from build123d import *

# Parameters (mm, degrees)
SKETCH_1_R = 1.5875


with BuildPart() as part:
    # 草图1 → 旋转1 (revolve)
    with BuildSketch(Plane.XY, mode=Mode.PRIVATE) as revolve_1_sk:
        with BuildLine():
            Line((42.275, 6.35), (42.275, 4.407946167))
            ThreePointArc((42.275, 4.407946167), (42.708118322, 3.857882219), (42.8625, 3.175))
            ThreePointArc((42.8625, 3.175), (42.708118322, 2.492117781), (42.275, 1.942053833))
            Line((42.275, 1.942053833), (42.275, 0))
            Line((42.275, 0), (44.45, 0))
            Line((44.45, 0), (44.45, 6.1))
            Line((44.45, 6.1), (44.45, 6.35))
            Line((44.45, 6.35), (42.275, 6.35))
        make_face()
        with BuildLine():
            Line((40.275, 6.35), (38.1, 6.35))
            Line((38.1, 6.35), (38.1, 6.1))
            Line((38.1, 6.1), (38.1, 0))
            Line((38.1, 0), (40.275, 0))
            Line((40.275, 0), (40.275, 1.942053833))
            ThreePointArc((40.275, 1.942053833), (39.6875, 3.175), (40.275, 4.407946167))
            Line((40.275, 4.407946167), (40.275, 6.35))
        make_face()
        with Locations((41.275, 3.175)):
            Circle(SKETCH_1_R)
    revolve(revolve_1_sk.sketch.rotate(Axis((0, 13.35, 0), (0, 1, 0)), 90), axis=Axis((0, 13.35, 0), (0, 1, 0)))


solid = part.part
The model under review builds one solid part; all positions refer to its coordinate system, in mm. Round coordinates to 2 decimals unless told otherwise and drop trailing zeros. Return JSON: item names as keys, results as strings.
(1) The part is to be moulded in two halves that separate along Z. For faces 1 (the cylindrical face through (-30, 3.2, 32.8)), 2 (the flat face through (30, 0, -24)), 3 (the cylindrical face through (-12.098, 5.393, -38.415)), say which applies: released by +Z, released by -Z, zero draft, split by the parting line, or undercut.
Solved:
{"face 1": "split by the parting line", "face 2": "zero draft", "face 3": "undercut"}
(2) For line 1 (X direction, y = 1.2, z = 0) (3 decimals); line 2 (X direction, y = 5.25, z = -4); line 3 (Z direction, x = 11, y = 1.5), list the stretches that pass through material, from the lowest coordinate up.
Solved:
{"line 1": "-44.45 to -42.275, -40.275 to -38.1, 38.1 to 40.275, 42.275 to 44.45", "line 2": "-44.27 to -42.09, -40.08 to -37.89, 37.89 to 40.08, 42.09 to 44.27", "line 3": "-43.07 to -40.82, -38.74 to -36.48, 36.48 to 38.74, 40.82 to 43.07"}
(3) For pin 1 (1.5 mm diameter, centred on y = 0.5, z = 12.5, fed in from +X); pin 2 (2 mm diameter, centred on x = 13.5, y = 4.5, fed in from +Z); pin 3 (1.5 mm diameter, centred on x = -23.5, y = 2, fed in from +Z), all flat-tipped, find the tip position at first contact; note any pin that passes through.
Solved:
{"pin 1": "x = 42.87", "pin 2": "z = 42.66", "pin 3": "z = 38.19"}
